from build123d import *

# Parameters (mm, degrees)
ESQUISSE1_R        = 10
ESQUISSE1_R_2      = 0.6
BOSS_EXTRU_1_DEPTH = 4
ESQUISSE3_R        = 5
BOSS_EXTRU_2_DEPTH = 5
ESQUISSE4_W        = 8
ESQUISSE4_H        = 38
BOSS_EXTRU_3_DEPTH = 2


with BuildPart() as part:
    # Esquisse1 → Boss.-Extru.1 (new body)
    with BuildSketch(Plane.XY):
        Circle(ESQUISSE1_R)
        with Locations((0, -7.5)):
            Circle(ESQUISSE1_R_2, mode=Mode.SUBTRACT)
        with Locations((0, 7.5)):
            Circle(ESQUISSE1_R_2, mode=Mode.SUBTRACT)
    extrude(amount=BOSS_EXTRU_1_DEPTH)

    # Esquisse3 → Boss.-Extru.2 (add)
    with BuildSketch(Plane.XY.offset(4)):
        Circle(ESQUISSE3_R)
        with BuildLine():
            Line((-2.142428529, 2.1), (2.142428529, 2.1))
            ThreePointArc((2.142428529, 2.1), (0, -3), (-2.142428529, 2.1))
        make_face(mode=Mode.SUBTRACT)
    extrude(amount=BOSS_EXTRU_2_DEPTH)

    # Esquisse4 → Boss.-Extru.3 (add)
    with BuildSketch(Plane(origin=(0, 0, 0), x_dir=(-1, 0, 0), z_dir=(0, 0, -1))):
        Rectangle(ESQUISSE4_W, ESQUISSE4_H)
    extrude(amount=BOSS_EXTRU_3_DEPTH)


solid = part.part
Here's how the part is built. I have some questions about the finished solid (model axes, mm). A direction names the side the tool comes from. Round coordinates to 2 decimals unless told otherwise and drop trailing zeros. Loops run counter-clockwise (first coordinate to the right, second up) from the corner with the lowest first, then second, coordinate; pieces in that order, holes last. Notation, with made-up numbers: (13, -9.75) - (28, -9.75) arc R20 cw to (28, 6.25) - close; hole circle Ø11 at (37, -27). An arc over 180 degrees is marked (long way). One line per question, with ' | ' between items. Start each with the question number.
Q1. I want a section at A-A (x = 0). Write out the boundary of the cut face in (y, z).
Q2. Please list where these lines run through material, in increasing order: line 1 (Y direction, x = 0, z = 1.1); line 2 (Y direction, x = 0, z = 5.75); line 3 (Z direction, x = -3.25, y = -16.5). Write a range as [from, to].
Q3. Will these pins go through, and if not, where does the flat tip stop? pin 1 (3 mm diameter, centred on x = -7, y = -5.5, fed in from -Z); pin 2 (1.3 mm diameter, centred on x = -1, z = 7.5, fed in from -Y); pin 3 (9 mm diameter, centred on x = -1.5, y = 15.5, fed in from +Z); pin 4 (5 mm diameter, centred on y = 11, z = 7, fed in from -X).
Q4. For faces 1 (the flat face through (-6, 0, 0)), 2 (the flat face through (-5, -2, 4)), 3 (the flat face through (4, 0, -1)), which set-ups out of +Z, -Z, +X, -X, +Y, -Y let a thin tool reach every point of the face, with its end or its side?
Q5. I want a section at B-B (y = 0). Write out the boundary of the cut face in (x, z), then the cut area to 3 significant figures.
Q6. I want a section at C-C (z = 3.5). Write out the boundary of the cut face in (x, y).
Q7. I want a section at D-D (z = 5.5). Write out the boundary of the cut face in (x, y), then the cut area to 3 significant figures.
Response values:
1) outline: (-19, -2) - (19, -2) - (19, 0) - (10, 0) - (10, 4) - (8.1, 4) - (8.1, 0) - (6.9, 0) - (6.9, 4) - (5, 4) - (5, 9) - (2.1, 9) - (2.1, 4) - (-3, 4) - (-3, 9) - (-5, 9) - (-5, 4) - (-6.9, 4) - (-6.9, 0) - (-8.1, 0) - (-8.1, 4) - (-10, 4) - (-10, 0) - (-19, 0) - close
2) line 1: y = [-10, -8.1], [-6.9, 6.9], [8.1, 10] | line 2: y = [-5, -3], [2.1, 5] | line 3: z = [-2, 0]
3) pin 1: stops at z = 0 | pin 2: stops at y = -4.99 | pin 3: stops at z = 0 | pin 4: passes through
4) face 1: -Z, -X, +Y, -Y | face 2: +Z | face 3: -Z, +X, +Y, -Y
5) outline: (-10, 0) - (-4, 0) - (-4, -2) - (4, -2) - (4, 0) - (10, 0) - (10, 4) - (5, 4) - (5, 9) - (3, 9) - (3, 4) - (-3, 4) - (-3, 9) - (-5, 9) - (-5, 4) - (-10, 4) - close | area: 116 mm²
6) outline: circle Ø20 at (0, 0); hole circle Ø1.2 at (0, -7.5); hole circle Ø1.2 at (0, 7.5)
7) outline: circle Ø10 at (0, 0); hole (-2.14, 2.1) arc R3 ccw (long way) to (2.14, 2.1) - close | area: 52.9 mm²
